Can you work these out from the model? Positions are in its coordinate system, mm. Give positions to 0.01 mm unless a question says otherwise; leave off trailing zeros. Order: outer loops, then holes, each group sorted by start corner. A loop starts at its lowest first (then second) coordinate and runs counter-clockwise, first axis right, second up.
Item 1: I want a section at B-B, the plane z = -1.45. Write out the boundary of the cut face in (x, y), then the cut area to 3 significant figures.
Item 2: I want a section at A-A, the plane x = 89.5. Write out the boundary of the cut face in (y, z), then the cut area to 3 significant figures.
Item 3: I'm going to push flat-ended pins straight in: pin 1 Ø1.5 at (x, z) = (15, -1.5) entering from +Y; pin 2 Ø1 at (x, z) = (79.5, -1.5) entering from +Y. Where does each tip first touch, or does it pass through?
Item 4: If I drill on line 1 along Y through (x, z) = (67, -1.65); line 2 along Y through (x, z) = (104.5, -1.45); line 3 along Z through (x, y) = (122, 1.75), over which ranges is the centre line in solid material (lowest first)?
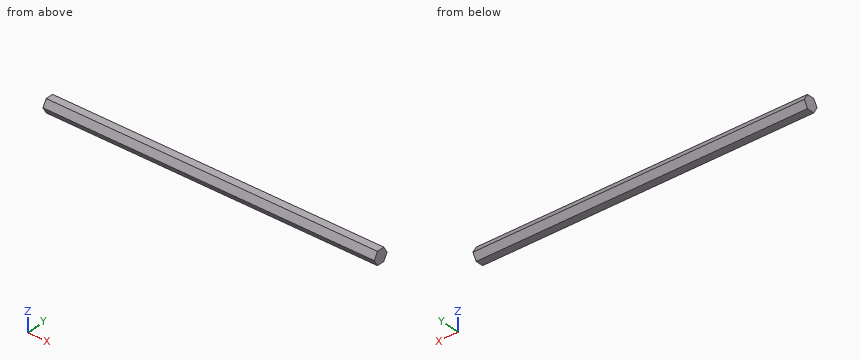
Autodesk Inventor part; units mm, degrees
ref_plane "YZ Plane" through (0, 0, 0) normal (1, 0, 0) x (0, 1, 0)
ref_plane "XZ Plane" through (0, 0, 0) normal (0, 1, 0) x (-1, 0, 0)
ref_plane "XY Plane" through (0, 0, 0) normal (0, 0, 1) x (1, 0, 0)
sketch "Sketch1" plane through (0, 0, 0) normal (1, 0, 0) x (0, 1, 0)
  line L0 (-1.5584, 2.6992) -> (-3.1168, 0)
  line L1 (1.5584, 2.6992) -> (-1.5584, 2.6992)
  line L2 (3.1168, 0) -> (1.5584, 2.6992)
  line L3 (1.5584, -2.6992) -> (3.1168, 0)
  line L4 (-1.5584, -2.6992) -> (1.5584, -2.6992)
  line L5 (-3.1168, 0) -> (-1.5584, -2.6992)
  point P0 (0, 0)
  point P1 (0, 0)
  point P2 (0, 0)
extrude "Extrusion1" add sketch "Sketch1" along normal blind 134.9375
sketch "Sketch2" plane through (0, 0, 0) normal (-1, 0, 0) x (0, 0, 1)
  point P0 (0, 0)
  point P1 (0, 0)
sketch "Sketch3" plane through (134.9375, 0, 0) normal (1, 0, 0) x (0, 0, -1)
  point P0 (0, 0)
  point P1 (0, 0)
properties part number "HexShaft"
Results list:
1. outline: (0, -2.28) - (134.94, -2.28) - (134.94, 2.28) - (0, 2.28) - close
1. area: 615 mm2
2. outline: (-3.12, 0) - (-1.56, -2.7) - (1.56, -2.7) - (3.12, 0) - (1.56, 2.7) - (-1.56, 2.7) - close
2. area: 25.2 mm2
3. pin 1: stops at y = 2.68
3. pin 2: stops at y = 2.54
4. line 1: y = -2.16 to 2.16
4. line 2: y = -2.28 to 2.28
4. line 3: z = -2.37 to 2.37
